Work out the finished part from the listing and answer in its coordinate system (mm). Coordinates: 2 decimals unless noted, no trailing zeros. Order: outer loops, then holes, each group sorted by start corner. A loop starts at its lowest first (then second) coordinate and runs counter-clockwise, first axis right, second up. Notation, with made-up numbers: (76.25, 24.5) - (128.25, 24.5) arc R35 ccw to (128.25, 59.5) - close; hole circle Ø6 at (25, -1.75). An arc over 180 degrees is marked (long way). Answer as a JSON object with one key per item and string values. Group by question number.
1) Section C-C (z = 1.25) is taken. Give the vertices of the cut face in (x, y), plus the area to 3 significant figures.
2) Section B-B (y = 5.75) is taken. Give the vertices of the cut face in (x, z), plus the area to 3 significant figures.
3) Find the intervals of material crossed by line 1 along X through (y, z) = (5.7, -15); line 2 along Y through (x, z) = (1, -10); line 3 along Z through (x, y) = (0.75, 2), in increasing order.
4) Each of these flat-tipped pins is pushed along its axis until it touches: P1, Ø2, axis at x = 1, z = -3, coming from the -Y side; P2, Ø2, axis at y = 4, z = 0, coming from the -X side; P3, Ø3, axis at y = 1.5, z = 1, coming from the -X side. Where does it stop, or does it pass through?
5) Section A-A (x = 0) is taken. Give the vertices of the cut face in (y, z), plus the area to 3 significant figures.
6) The mould has two halves that part along Z. Classify faces 1 (the face through (-2, 2, 0)), 2 (the face through (0, 0, 0)), 3 (the face through (-0.632, 5.49, -13.476)): released by +Z, released by -Z, zero draft, split by the parting line, or undercut.
7) Section D-D (y = 3.25) is taken. Give the vertices of the cut face in (x, z).
from build123d import *

# Parameters (mm, degrees)
SKETCH_1_R      = 2
EXTRUDE_1_DEPTH = 4.8
SKETCH_2_R      = 1.65
EXTRUDE_2_DEPTH = 1.4


with BuildPart() as part:
    # 草图1 → 凸台-拉伸1 (new body)
    with BuildSketch(Plane(origin=(0, 0, 0), x_dir=(1, 0, 0), z_dir=(0, 1, 0))):
        with Locations(Location((0, 0, 0), (0, 0, 270))):
            Circle(SKETCH_1_R)
    extrude(amount=EXTRUDE_1_DEPTH)

    # 草图2 → 凸台-拉伸2 (add)
    with BuildSketch(Plane(origin=(0, 4.8, 0), x_dir=(1, 0, 0), z_dir=(0, 1, 0))):
        with BuildLine():
            Line((-3.5, 0), (-3.5, 15))
            ThreePointArc((-3.5, 15), (0, 18.5), (3.5, 15))
            Line((3.5, 15), (3.5, 0))
            ThreePointArc((3.5, 0), (0, -3.5), (-3.5, 0))
        make_face()
        with Locations(Location((0, 15, 0), (0, 0, 270))):
            Circle(SKETCH_2_R, mode=Mode.SUBTRACT)
    extrude(amount=EXTRUDE_2_DEPTH)


solid = part.part
Report:
{
 "1": {"outline": "(-3.27, 4.8) - (-1.56, 4.8) - (-1.56, 0) - (1.56, 0) - (1.56, 4.8) - (3.27, 4.8) - (3.27, 6.2) - (-3.27, 6.2) - close", "area": "24.1 mm²"},
 "2": {"outline": "(-3.5, -15) arc R3.5 ccw to (3.5, -15) - (3.5, 0) arc R3.5 ccw to (-3.5, 0) - close; hole circle Ø3.3 at (0, -15)", "area": "135 mm²"},
 "3": {"line 1": "x = -3.5 to -1.65, 1.65 to 3.5", "line 2": "y = 4.8 to 6.2", "line 3": "z = -1.85 to 1.85"},
 "4": {"P1": "stops at y = 4.8", "P2": "stops at x = -3.5", "P3": "stops at x = -2"},
 "5": {"outline": "(0, -2) - (4.8, -2) - (4.8, -13.35) - (6.2, -13.35) - (6.2, 3.5) - (4.8, 3.5) - (4.8, 2) - (0, 2) - close; (4.8, -18.5) - (6.2, -18.5) - (6.2, -16.65) - (4.8, -16.65) - close", "area": "45.4 mm²"},
 "6": {"face 1": "split by the parting line", "face 2": "zero draft", "face 3": "undercut"},
 "7": {"outline": "circle Ø4 at (0, 0)"}
}
